from build123d import *

# Parameters (mm, degrees)
SKETCH_1_R               = 148.1
SKETCH_1_R_2             = 125
EXTRUDE_1_DEPTH          = 12
SKETCH_2_R               = 142.1
SKETCH_2_R_2             = 125
EXTRUDE_2_DEPTH          = 6
SKETCH_3_R               = 148.1
SKETCH_3_R_2             = 125
EXTRUDE_3_DEPTH          = 5
SKETCH_4_R               = 133.1
SKETCH_4_R_2             = 125
EXTRUDE_4_DEPTH          = 10
SKETCH_5_R               = 148.1
SKETCH_5_R_2             = 125
EXTRUDE_5_DEPTH          = 5
SKETCH_6_R               = 2
EXTRUDE_6_DEPTH          = 12
SKETCH_7_R               = 2.5
CUT_EXTRUDE_1_DEPTH      = 15
MIRROR_2_COPY_1_SKETCH_R = 2.5
MIRROR_2_COPY_1_DEPTH    = 15
CHAMFER_1_SIZE           = 5


with BuildPart() as part:
    # 草图1 → 凸台-拉伸1 (new body)
    with BuildSketch(Plane.XY):
        Circle(SKETCH_1_R)
        Circle(SKETCH_1_R_2, mode=Mode.SUBTRACT)
    extrude(amount=EXTRUDE_1_DEPTH)

    # 草图2 → 凸台-拉伸2 (add)
    with BuildSketch(Plane.XY.offset(12)):
        Circle(SKETCH_2_R)
        Circle(SKETCH_2_R_2, mode=Mode.SUBTRACT)
    extrude(amount=EXTRUDE_2_DEPTH)

    # 草图3 → 凸台-拉伸3 (add)
    with BuildSketch(Plane.XY.offset(18)):
        Circle(SKETCH_3_R)
        Circle(SKETCH_3_R_2, mode=Mode.SUBTRACT)
    extrude(amount=EXTRUDE_3_DEPTH)

    # 草图4 → 凸台-拉伸4 (add)
    with BuildSketch(Plane.XY.offset(23)):
        Circle(SKETCH_4_R)
        Circle(SKETCH_4_R_2, mode=Mode.SUBTRACT)
    extrude(amount=EXTRUDE_4_DEPTH)

    # 草图5 → 凸台-拉伸5 (add)
    with BuildSketch(Plane.XY.offset(33)):
        Circle(SKETCH_5_R)
        Circle(SKETCH_5_R_2, mode=Mode.SUBTRACT)
    extrude(amount=EXTRUDE_5_DEPTH)

    # 草图6 → 凸台-拉伸6 (add)
    # profile 1 of 4: a face of its own
    with BuildSketch(Plane.XY):
        with BuildLine():
            Line((-90.799834802, 117), (-110.208193805, 117))
            ThreePointArc((-110.208193805, 117), (-117.683675787, 111.849064607), (-115.532726589, 103.029292284))
            Line((-115.532726589, 103.029292284), (-110.532726589, 98.570413171))
            ThreePointArc((-110.532726589, 98.570413171), (-101.087152926, 108.235842092), (-90.799834802, 117))
        make_face()
        with Locations((-110.208193805, 109)):
            Circle(SKETCH_6_R, mode=Mode.SUBTRACT)
    # profile 2 of 4: a face of its own
    with BuildSketch(Plane.XY):
        with BuildLine():
            Line((115.532726589, 103.029292284), (110.532726589, 98.570413171))
            ThreePointArc((110.532726589, 98.570413171), (101.087152926, 108.235842092), (90.799834802, 117))
            Line((90.799834802, 117), (110.208193805, 117))
            ThreePointArc((110.208193805, 117), (117.683675787, 111.849064607), (115.532726589, 103.029292284))
        make_face()
        with Locations(Location((110.208193805, 109, 0), (0, 0, 180))):
            Circle(SKETCH_6_R, mode=Mode.SUBTRACT)
    # profile 3 of 4: a face of its own
    with BuildSketch(Plane.XY):
        with BuildLine():
            Line((115.532726589, -103.029292284), (110.532726589, -98.570413171))
            ThreePointArc((110.532726589, -98.570413171), (101.087152926, -108.235842092), (90.799834802, -117))
            Line((90.799834802, -117), (110.208193805, -117))
            ThreePointArc((110.208193805, -117), (117.683675787, -111.849064607), (115.532726589, -103.029292284))
        make_face()
        with Locations((110.208193805, -109)):
            Circle(SKETCH_6_R, mode=Mode.SUBTRACT)
    # profile 4 of 4: a face of its own
    with BuildSketch(Plane.XY):
        with BuildLine():
            Line((-115.532726589, -103.029292284), (-110.532726589, -98.570413171))
            ThreePointArc((-110.532726589, -98.570413171), (-101.087152926, -108.235842092), (-90.799834802, -117))
            Line((-90.799834802, -117), (-110.208193805, -117))
            ThreePointArc((-110.208193805, -117), (-117.683675787, -111.849064607), (-115.532726589, -103.029292284))
        make_face()
        with Locations(Location((-110.208193805, -109, 0), (0, 0, 180))):
            Circle(SKETCH_6_R, mode=Mode.SUBTRACT)
    extrude(amount=EXTRUDE_6_DEPTH)

    # 草图7 → 切除-拉伸1 (cut)
    with BuildSketch(Plane(origin=(0, 117, 0), x_dir=(1, 0, 0), z_dir=(0, 1, 0))):
        with Locations(Location((-98.799834802, -6, 0), (0, 0, 270))):
            Circle(SKETCH_7_R)
    cut_extrude_1 = extrude(amount=-CUT_EXTRUDE_1_DEPTH, mode=Mode.SUBTRACT)

    # 镜向1: 切除-拉伸1 across plane
    add(cut_extrude_1.mirror(Plane(origin=(0, 0, 0), x_dir=(0, 0, 1), z_dir=(1, 0, 0))), mode=Mode.SUBTRACT)

    # 镜向2: 切除-拉伸1 across plane
    add(cut_extrude_1.mirror(Plane.ZX), mode=Mode.SUBTRACT)

    # 镜向2 copy 1 sketch → 镜向2 copy 1 (cut)
    with BuildSketch(Plane(origin=(0, -117, 0), x_dir=(-1, 0, 0), z_dir=(0, -1, 0))):
        with Locations(Location((-98.799834802, -6, 0), (0, 0, 270))):
            Circle(MIRROR_2_COPY_1_SKETCH_R)
    extrude(amount=-MIRROR_2_COPY_1_DEPTH, mode=Mode.SUBTRACT)

    # 倒角1
    chamfer_1_edges = [part.edges().sort_by_distance(p)[0] for p in [
        (-125, 0, 0),
    ]]
    chamfer(chamfer_1_edges, length=CHAMFER_1_SIZE)


solid = part.part
Can you work these out from the model? Positions are in its coordinate system, mm. A direction names the side the tool comes from. Round coordinates to 2 decimals unless told otherwise and drop trailing zeros. Order: outer loops, then holes, each group sorted by start corner. A loop starts at its lowest first (then second) coordinate and runs counter-clockwise, first axis right, second up. Notation, with made-up numbers: M 85.5,69 L 100.5,69 A18 cw 100.5,95 Z; hole C 46,-9 d7. An arc over 180 degrees is marked long. Use a Markdown table: item, result.
1) On a 3-axis mill with a long thin cutter (end or side, diameter ignored), from which of +Z, -Z, +X, -X, +Y, -Y can I reach the whole of each face in a straight line? I mean faces 1 (the face through (-77, 121, 12)), 2 (the face through (-103, -117, 6)), 3 (the face through (103, 117, 6)). Say none if no direction works.
Geometry says:
| item | result |
|---|---|
| face 1 | none |
| face 2 | +Z, -Z, -X, -Y |
| face 3 | +Z, -Z, +X, +Y |
2) I'm going to push flat-ended pins straight in: P1, Ø1.5, axis at y = 54.5, z = 9.5, coming from the -X side; P2, Ø1, axis at x = -71, z = 29, coming from the +Y side; P3, Ø9.5, axis at x = -101.5, z = 6.5, coming from the +Y side; P4, Ø2.5, axis at x = 110.21, y = 109, coming from the -Z side. Where does each tip first touch, or does it pass through?
Geometry says:
| item | result |
|---|---|
| P1 | stops at x = -138 |
| P2 | stops at y = 112.9 |
| P3 | stops at y = 117 |
| P4 | passes through |
3) Imagine slicing it at A-A (y = 0). List the corners of the cut face in (x, z) for me.
Geometry says:
| item | result |
|---|---|
| outline | M -148.1,0 L -130,0 L -125,5 L -125,38 L -148.1,38 L -148.1,33 L -133.1,33 L -133.1,23 L -148.1,23 L -148.1,18 L -142.1,18 L -142.1,12 L -148.1,12 Z; M 125,5 L 130,0 L 148.1,0 L 148.1,12 L 142.1,12 L 142.1,18 L 148.1,18 L 148.1,23 L 133.1,23 L 133.1,33 L 148.1,33 L 148.1,38 L 125,38 Z |
4) If we mould it in two halves opening along Y, with no side actions, what happens to faces 4 (the face through (117.634, 111.975, 5.916)), 5 (the face through (10, 132, 0)), 6 (the face through (-117.634, -111.975, 5.916)), 7 (the face through (1.368, 148.094, 5.916))? For each: +Y half, -Y half, draft (parallel to the pull), parting line (faces both ways), or undercut.
Geometry says:
| item | result |
|---|---|
| face 4 | undercut |
| face 5 | draft |
| face 6 | undercut |
| face 7 | +Y half |
5) If I drill on line 1 along X through (y, z) = (-54, 7); line 2 along X through (y, z) = (63, 22); line 3 along Y through (x, z) = (-92.5, 34), over which ranges is the centre line in solid material (lowest first)?
Geometry says:
| item | result |
|---|---|
| line 1 | x = -137.9 to -112.73, 112.73 to 137.9 |
| line 2 | x = -134.03 to -107.96, 107.96 to 134.03 |
| line 3 | y = -115.66 to -84.08, 84.08 to 115.66 |
